from build123d import *

# Parameters (mm, degrees)
SKETCH_1_R          = 12
EXTRUDE_1_DEPTH     = 11
EXTRUDE_START       = -11
SKETCH_2_R          = 3
EXTRUDE_2_DEPTH     = 20
SKETCH_3_W          = 68
SKETCH_3_H          = 37
EXTRUDE_3_DEPTH     = 1.1
SKETCH_3_3_R        = 13.15
EXTRUDE_4_DEPTH     = 11
CUT_EXTRUDE_START   = -2.5
SKETCH_5_R          = 13.15
SKETCH_5_R_2        = 10
CUT_EXTRUDE_2_DEPTH = 2.5
EXTRUDE_START_2     = -1.1
SKETCH_6_R          = 11.8
EXTRUDE_5_DEPTH     = 6.5
SKETCH_6_3_R        = 13.5
EXTRUDE_6_DEPTH     = 4.2
SKETCH_6_4_R        = 3.05
EXTRUDE_7_DEPTH     = 8.8
SKETCH_4_R          = 1.5
SKETCH_4_R_2        = 1.1
CUT_EXTRUDE_1_DEPTH = 61.205149281
SKETCH_7_R          = 1.25
CUT_EXTRUDE_3_DEPTH = 2.5


with BuildPart() as part:
    # 草图1 → 凸台-拉伸1 (new body)
    with BuildSketch(Plane.XY):
        Circle(SKETCH_1_R)
    extrude(amount=EXTRUDE_1_DEPTH)

    # 草图2 → 凸台-拉伸2 (add)
    with BuildSketch(Plane(origin=(0, 0, 0), x_dir=(-1, 0, 0), z_dir=(0, 0, -1)).offset(EXTRUDE_START)):
        with Locations(Location((0, 0, 0), (0, 0, 180))):
            Circle(SKETCH_2_R)
    extrude(amount=EXTRUDE_2_DEPTH)

    # 草图3 → 凸台-拉伸3 (add)
    with BuildSketch(Plane.XY):
        with Locations((22, 0)):
            Rectangle(SKETCH_3_W, SKETCH_3_H)
    extrude(amount=-EXTRUDE_3_DEPTH)

    # 草图3<3> → 凸台-拉伸4 (add)
    with BuildSketch(Plane.XY):
        with Locations((42.6, 0)):
            Circle(SKETCH_3_3_R)
    extrude(amount=-EXTRUDE_4_DEPTH)

    # 草图5 → 切除-拉伸2 (cut)
    with BuildSketch(Plane(origin=(0, 0, -11), x_dir=(-1, 0, 0), z_dir=(0, 0, -1)).offset(CUT_EXTRUDE_START)):
        with Locations(Location((-42.6, 0, 0), (0, 0, 180))):
            Circle(SKETCH_5_R)
        with Locations((-42.6, 0)):
            Circle(SKETCH_5_R_2, mode=Mode.SUBTRACT)
    extrude(amount=CUT_EXTRUDE_2_DEPTH, mode=Mode.SUBTRACT)

    # 草图6 → 凸台-拉伸5 (add)
    with BuildSketch(Plane(origin=(0, 0, -1.1), x_dir=(-1, 0, 0), z_dir=(0, 0, -1)).offset(EXTRUDE_START_2)):
        with Locations((-13.5, 3.6)):
            Circle(SKETCH_6_R)
    extrude(amount=EXTRUDE_5_DEPTH)

    # 草图6<3> → 凸台-拉伸6 (add)
    with BuildSketch(Plane(origin=(0, 0, -1.1), x_dir=(-1, 0, 0), z_dir=(0, 0, -1)).offset(EXTRUDE_START_2)):
        with Locations((-26.7, -2.2)):
            Circle(SKETCH_6_3_R)
    extrude(amount=EXTRUDE_6_DEPTH)

    # 草图6<4> → 凸台-拉伸7 (add)
    with BuildSketch(Plane(origin=(0, 0, -1.1), x_dir=(-1, 0, 0), z_dir=(0, 0, -1)).offset(EXTRUDE_START_2)):
        with Locations(Location((-26.7, -2.2, 0), (0, 0, 180))):
            Circle(SKETCH_6_4_R)
    extrude(amount=EXTRUDE_7_DEPTH)

    # 草图4 → 切除-拉伸1 (cut, through all)
    with BuildSketch(Plane(origin=(0, 0, -1.1), x_dir=(-1, 0, 0), z_dir=(0, 0, -1))):
        with Locations((1.9, 14.7)):
            Circle(SKETCH_4_R)
        with Locations((1.9, -14.7)):
            Circle(SKETCH_4_R)
        with Locations((-35.9, 15.4)):
            Circle(SKETCH_4_R_2)
        with Locations((-35.9, -15.4)):
            Circle(SKETCH_4_R_2)
    extrude(amount=-CUT_EXTRUDE_1_DEPTH, mode=Mode.SUBTRACT)

    # 草图7 → 切除-拉伸3 (cut)
    with BuildSketch(Plane(origin=(0, 0, -11), x_dir=(-1, 0, 0), z_dir=(0, 0, -1))):
        with Locations((-48.85, 0)):
            Circle(SKETCH_7_R)
        with Locations((-36.35, 0)):
            Circle(SKETCH_7_R)
    extrude(amount=-CUT_EXTRUDE_3_DEPTH, mode=Mode.SUBTRACT)


solid = part.part
Work out the finished part from the listing and answer in its coordinate system (mm). A direction names the side the tool comes from. Coordinates: 2 decimals unless noted, no trailing zeros. Write each loop counter-clockwise with the first axis right and the second up, starting at its lowest first coordinate (ties: lowest second). Pieces come first, ordered by that corner, then holes. Notation, with made-up numbers: M 26,26.25 L 67,26.25 A13 cw 67,48.25 Z; hole C 52,29 d9. An arc over 180 degrees is marked long. Use one line per item in the form item = value. Start each with the question number.
1. A tool of negligible diameter and unlimited length cuts with its end or side. For faces 1 (the face through (-11.99, 0.53, 5.42)), 2 (the face through (52.59, 0.44, -9.73)), 3 (the face through (24.77, -15.56, -2.63)), 4 (the face through (0, 0, -9)), 5 (the face through (28.24, 11.21, -2.63)), from which of +Z, -Z, +X, -X, +Y, -Y can it reach the whole face along a straight path? Write none if from no direction.
2. The part is cut by section D-D (z = -3). Give the vertices of the cut face in (x, y).
3. Each of these flat-tipped pins is pushed along its axis until it touches: P1, Ø4, axis at x = 28, y = -12, coming from the -Z side; P2, Ø1.8, axis at x = -0.5, y = -1, coming from the -Z side; P3, Ø3, axis at x = 27.5, y = -1.5, coming from the -Z side. Where does it stop, or does it pass through?
4. The part is cut by section B-B (x = -1.9). Give the vertices of the cut face in (y, z).
5. The part is cut by section A-A (x = 26.7). Give the vertices of the cut face in (y, z), plus the area to 3 significant figures.
6. The part is cut by section C-C (x = 42.6). Give the vertices of the cut face in (y, z), plus the area to 3 significant figures.
7. Straight lines are drawn through the part: probe 1 along Y at (x, z) = (35.9, -0.75); probe 2 along Z at (x, y) = (32, -12); probe 3 along Z at (x, y) = (2, 17). For each, find the intervals that lie inside material, in ascending order. Write a range as from..to.
Evaluation:
q1.face_1 = +Z
q1.face_2 = -Z
q1.face_3 = -Z, -Y
q1.face_4 = -Z, -X, +Y, -Y
q1.face_5 = -Z, +Y
q2.outline = M 1.76,2.43 A3 ccw long 2.74,-1.23 A11.8 ccw 14.58,-8.15 A13.5 ccw 36.4,-11.59 A13.15 ccw long 33.48,9.47 A13.5 ccw 22.89,10.75 A11.8 ccw Z
q3.P1 = -4.2
q3.P2 = -9
q3.P3 = -8.8
q4.outline = M -18.5,-1.1 L -16.2,-1.1 L -16.2,0 L -18.5,0 Z; M -13.2,-1.1 L -2.32,-1.1 L -2.32,-9 L 2.32,-9 L 2.32,-1.1 L 13.2,-1.1 L 13.2,0 L 11.85,0 L 11.85,11 L -11.85,11 L -11.85,0 L -13.2,0 Z; M 16.2,-1.1 L 18.5,-1.1 L 18.5,0 L 16.2,0 Z
q5.outline = M -18.5,-1.1 L -15.7,-1.1 L -15.7,-4.2 L -5.25,-4.2 L -5.25,-8.8 L 0.85,-8.8 L 0.85,-4.2 L 11.3,-4.2 L 11.3,-1.1 L 18.5,-1.1 L 18.5,0 L -18.5,0 Z
q5.area = 152 mm^2
q6.outline = M -18.5,-1.1 L -13.15,-1.1 L -13.15,-8.5 L -10,-8.5 L -10,-11 L 10,-11 L 10,-8.5 L 13.15,-8.5 L 13.15,-1.1 L 18.5,-1.1 L 18.5,0 L -18.5,0 Z
q6.area = 285 mm^2
q7.probe_1 = -18.5..-16.5, -14.3..14.3, 16.5..18.5
q7.probe_2 = -4.2..0
q7.probe_3 = -1.1..0
